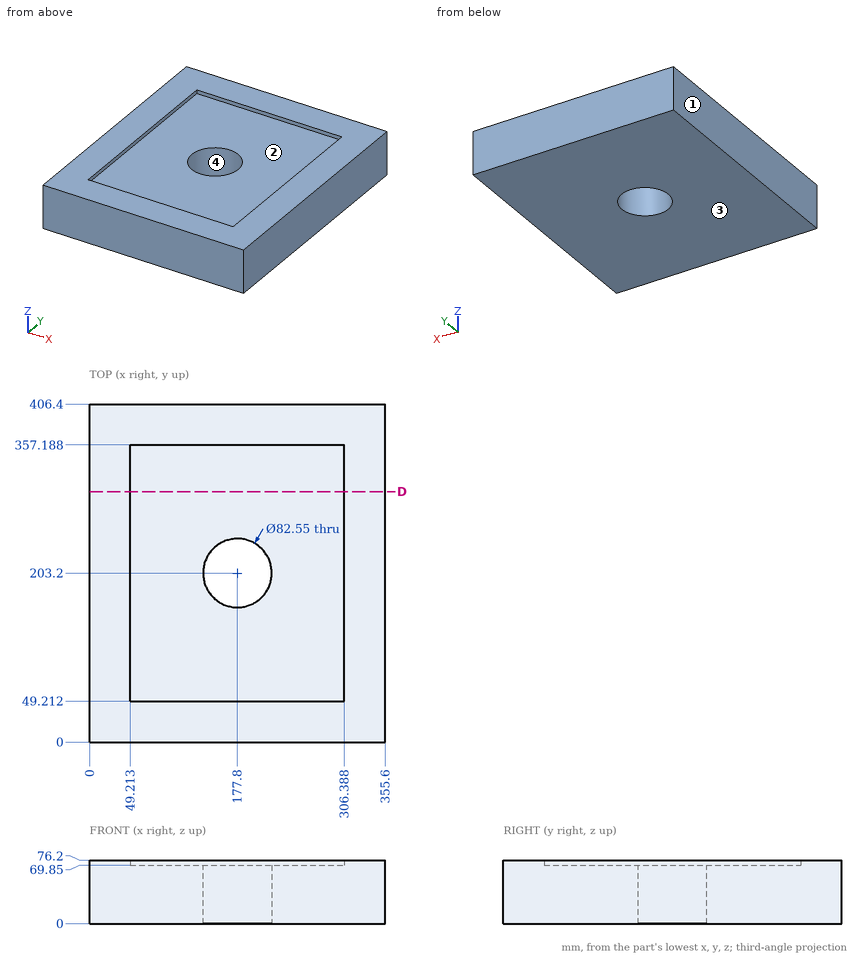
Can you work these out from the drawing? Everything is in mm from the part's minimum corner. Round coordinates to 2 decimals unless told otherwise and drop trailing zeros. Write each loop counter-clockwise with the first axis right and the second up, starting at its lowest first coordinate (ties: lowest second). Pieces come first, ordered by that corner, then holes.
1. Suppose I cut it at D-D (y = 301). List the corners of the cut face in (x, z) for me, and give its area (3 significant figures).
2. I need wall thicknesses on L1, parallel to Y at x = 177, z = 34; L2, parallel to Z at x = 110, y = 50.5; L3, parallel to X at y = 170, z = 9 (1 decimal). Which ranges of each line are inside material? Lowest first, please.
3. If we mould it in two halves opening along X, with no side actions, what happens to the marked faces 1, 2, 3 and 4? For each: released by +X, released by -X, zero draft, split by the parting line, or undercut.
4. Will this pin go through, and if not, where does the flat tip stop? pin 1 Ø5 at (x, y) = (69, 152.5) entering from +Z.
Answer sheet:
1. outline: (0, 0) - (355.6, 0) - (355.6, 76.2) - (306.39, 76.2) - (306.39, 69.85) - (49.21, 69.85) - (49.21, 76.2) - (0, 76.2) - close
1. area: 25,500 mm2
2. L1: y = 0 to 161.93, 244.47 to 406.4
2. L2: z = 0 to 69.85
2. L3: x = 0 to 153.3, 202.3 to 355.6
3. face 1: released by -X
3. face 2: undercut
3. face 3: zero draft
3. face 4: undercut
4. pin 1: stops at z = 69.85
